Could you check a few things on this model? Use its own coordinates, in mm. A direction names the side the tool comes from. Coordinates: 2 decimals unless noted, no trailing zeros. Loops run counter-clockwise (first coordinate to the right, second up) from the corner with the lowest first, then second, coordinate; pieces in that order, holes last.
from build123d import *

# Parameters (mm, degrees)
BOSS_EXTRUDE1_DEPTH     = 13.15
CUT_EXTRUDE2_DEPTH      = 14.892246039
CUT_EXTRUDE2_DEPTH_BACK = 13
SKETCH2_OUTSIDE_W       = 17.928
SKETCH2_OUTSIDE_H       = 7.018


with BuildPart() as part:
    # Sketch1 → Boss-Extrude1 (new body)
    with BuildSketch(Plane(origin=(0, 0, 0), x_dir=(0, 0, -1), z_dir=(1, 0, 0))):
        with BuildLine():
            Line((0, 0), (0.24, 0))
            ThreePointArc((0.24, 0), (0.421575008, 1.227565185), (0.9507497, 2.35))
            Line((0.9507497, 2.35), (2.24, 2.35))
            Line((2.24, 2.35), (2.24, 2.59))
            Line((2.24, 2.59), (1.122898476, 2.59))
            ThreePointArc((1.122898476, 2.59), (1.636238533, 3.145094281), (2.24, 3.600198407))
            Line((2.24, 3.600198407), (2.24, 3.88))
            ThreePointArc((2.24, 3.88), (0.60020249, 2.240089284), (0, 0))
        make_face()
    extrude(amount=BOSS_EXTRUDE1_DEPTH)

    # Sketch2 outside → Cut-Extrude2 (cut, two sides: drawn at the far end of the back side and taken through both)
    with BuildSketch(Plane(origin=(0, 0, 0), x_dir=(1, 0, 0), z_dir=(0, 1, 0)).offset(-CUT_EXTRUDE2_DEPTH_BACK)):
        with Locations((6.575, 1.12)):
            Rectangle(SKETCH2_OUTSIDE_W, SKETCH2_OUTSIDE_H)
        Polygon((0.917192044, 3), (12.232807956, 3), (13.15, 0), (0, 0), align=None, mode=Mode.SUBTRACT)
    extrude(amount=CUT_EXTRUDE2_DEPTH + CUT_EXTRUDE2_DEPTH_BACK, mode=Mode.SUBTRACT)


solid = part.part
(1) I need wall thicknesses on probe 1 along Y at (x, z) = (3, -1.4); probe 2 along Y at (x, z) = (9.75, -1.95); probe 3 along Y at (x, z) = (9.75, -0.65). Which ranges of each line are inside material? Lowest first, please.
Answers:
probe 1: y = 2.35 to 2.59, 2.91 to 3.25
probe 2: y = 2.35 to 2.59, 3.4 to 3.7
probe 3: y = 1.82 to 2.32
(2) Imagine slicing it at C-C, the plane y = 1.3. Write out the boundary of the cut face in (x, z), and give its area (3 significant figures).
Answers:
outline: (0.06, -0.19) - (0.14, -0.44) - (13.01, -0.44) - (13.09, -0.19) - close
area: 3.26 mm2
(3) Imagine slicing it at D-D, the plane z = -0.8. Write out the boundary of the cut face in (x, y), and give its area (3 significant figures).
Answers:
outline: (0.24, 2.11) - (12.91, 2.11) - (12.91, 2.56) - (0.24, 2.56) - close
area: 5.68 mm2
(4) Imagine slicing it at A-A, the plane x = 5.5. Write out the boundary of the cut face in (y, z).
Answers:
outline: (0, -0.24) arc R4.24 cw to (2.35, -0.95) - (2.35, -2.24) - (2.59, -2.24) - (2.59, -1.12) arc R4.24 cw to (3.6, -2.24) - (3.88, -2.24) arc R4.48 ccw to (0, 0) - close
(5) Which directions (+Z, -Z, +X, -X, +Y, -Y) give clear straight access to the entire face, cutting with the end or side of a thin tool? Please do faces 1 (the face through (6, 2.59, -2)), 2 (the face through (6, 2.35, -2)), 3 (the face through (6.483, 2.268, -0.617)).
Answers:
face 1: -Z, +X, -X
face 2: -Z, +X, -X, -Y
face 3: +Z, +X, -X, +Y
(6) Imagine slicing it at B-B, the plane z = -1.75. Write out the boundary of the cut face in (x, y).
Answers:
outline: (0.54, 2.35) - (12.61, 2.35) - (12.61, 2.59) - (0.54, 2.59) - close; (0.54, 3.24) - (12.61, 3.24) - (12.61, 3.55) - (0.54, 3.55) - close
